Model file for the job. Use its own axes, mm. Face numbers are marked on the shaded views. A direction names the side the tool comes from. Round coordinates to 2 decimals unless told otherwise and drop trailing zeros. Loops run counter-clockwise (first coordinate to the right, second up) from the corner with the lowest first, then second, coordinate; pieces in that order, holes last. Notation, with made-up numbers: (-35, -7.75) -> (22, -7.75) arc R21 cw to (22, 30.25) -> close; hole circle Ø1 at (10, 75). An arc over 180 degrees is marked (long way). Use a Markdown table: item, result. Add a question column.
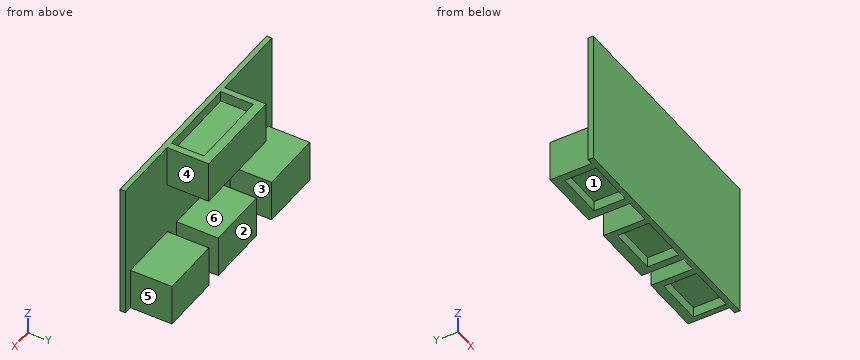
```python
from build123d import *

# Parameters (mm, degrees)
SKETCH1_W           = 23
SKETCH1_H           = 13
BOSS_EXTRUDE1_DEPTH = 0.5
SKETCH2_W           = 5.8
SKETCH2_H           = 4
SKETCH2_W_2         = 6
SKETCH2_W_3         = 9
BOSS_EXTRUDE2_DEPTH = 4
SKETCH3_W           = 4.624085026
SKETCH3_H           = 3.166867164
SKETCH3_W_2         = 4.718514666
SKETCH3_H_2         = 3.013327786
SKETCH3_W_3         = 4.580400568
CUT_EXTRUDE1_DEPTH  = 1
SKETCH4_W           = 7.748769295
SKETCH4_H           = 3.140290714
CUT_EXTRUDE2_DEPTH  = 1


with BuildPart() as part:
    # Sketch1 → Boss-Extrude1 (new body)
    with BuildSketch(Plane(origin=(0, 0, 0), x_dir=(1, 0, 0), z_dir=(0, 1, 0))):
        with Locations((1.517204559, 1.070232191)):
            Rectangle(SKETCH1_W, SKETCH1_H)
    extrude(amount=BOSS_EXTRUDE1_DEPTH)

    # Sketch2 → Boss-Extrude2 (add)
    with BuildSketch(Plane(origin=(0, 0.5, 0), x_dir=(1, 0, 0), z_dir=(0, 1, 0))):
        with Locations((9.339285907, 5.570232191)):
            Rectangle(SKETCH2_W, SKETCH2_H)
        with Locations((-6.403857402, 5.570232191)):
            Rectangle(SKETCH2_W_2, SKETCH2_H)
        with Locations((1.963830733, 5.570232191)):
            Rectangle(SKETCH2_W_2, SKETCH2_H)
        with Locations((1.962518624, -3.429767809)):
            Rectangle(SKETCH2_W_3, SKETCH2_H)
    extrude(amount=BOSS_EXTRUDE2_DEPTH)

    # Sketch3 → Cut-Extrude1 (cut)
    with BuildSketch(Plane(origin=(0, 0, -7.570232191), x_dir=(-1, 0, 0), z_dir=(0, 0, -1))):
        with Locations((-9.393748211, 2.083433582)):
            Rectangle(SKETCH3_W, SKETCH3_H)
        with Locations((-1.920682759, 2.006663893)):
            Rectangle(SKETCH3_W_2, SKETCH3_H_2)
        with Locations((6.437297708, 2.006663893)):
            Rectangle(SKETCH3_W_3, SKETCH3_H_2)
    extrude(amount=-CUT_EXTRUDE1_DEPTH, mode=Mode.SUBTRACT)

    # Sketch4 → Cut-Extrude2 (cut)
    with BuildSketch(Plane.XY.offset(5.429767809)):
        with Locations((1.929978032, 2.070145357)):
            Rectangle(SKETCH4_W, SKETCH4_H)
    extrude(amount=-CUT_EXTRUDE2_DEPTH, mode=Mode.SUBTRACT)


solid = part.part
```
1) Tool access for the marked faces 4, 5 and 6: list every direction of +Z, -Z, +X, -X, +Y, -Y with a clear straight run to the whole face (end or side of a thin tool).
2) Wall check: probe 1 along X at (y, z) = (1.25, -5.75); probe 2 along X at (y, z) = (1.35, -7); probe 3 along Z at (x, y) = (4, 0.75). Give the ranges that are in metal, low to high. Write a range as from..to.
3) Cut at D-D on z = 3.25. Write the cut outline in (x, y).
4) Pull direction Y, two halves, no side cores. Call the marked faces 1, 2 and 3: +Y half, -Y half, draft (parallel to the pull), parting line (faces both ways), or undercut.
5) Pin check, flat tips, straight feed: pin 1 Ø1.6 at (x, y) = (3, 2.5) entering from +Z; pin 2 Ø1.1 at (y, z) = (2, -7) entering from -X; pin 3 Ø0.5 at (y, z) = (1.5, -7) entering from +X. Stop position of each tip, or through.
6) Cut at C-C on y = 2.35. Count the separate pieces of the cut face and the enclosed holes in it, and give its area (3 significant figures).
7) Cut at B-B on x = 10.75. Write the cut outline in (y, z), and give its area (3 significant figures).
8) Cut at A-A on y = 4.05. Write the cut outline in (x, z).
Established:
| question | item | result |
|---|---|---|
| 1 | face 4 | +Z, +X, +Y |
| 1 | face 5 | +Z, -Z, +X, +Y |
| 1 | face 6 | +X, -X, +Y |
| 2 | probe 1 | x = -9.4..-3.4, -1.04..4.96, 6.44..12.24 |
| 2 | probe 2 | x = -9.4..-8.73, -4.15..-3.4, -1.04..-0.44, 4.28..4.96, 6.44..7.08, 11.71..12.24 |
| 2 | probe 3 | z = -6.57..-3.57, 1.43..4.43 |
| 3 | outline | (-9.98, 0) -> (13.02, 0) -> (13.02, 0.5) -> (6.46, 0.5) -> (6.46, 4.5) -> (-2.54, 4.5) -> (-2.54, 0.5) -> (-9.98, 0.5) -> close |
| 4 | face 1 | undercut |
| 4 | face 2 | +Y half |
| 4 | face 3 | draft |
| 5 | pin 1 | stops at z = 4.43 |
| 5 | pin 2 | stops at x = -9.4 |
| 5 | pin 3 | stops at x = 12.24 |
| 6 | separate pieces | 4 |
| 6 | enclosed holes | 0 |
| 6 | area | 85.5 mm^2 |
| 7 | outline | (0, -7.57) -> (0.5, -7.57) -> (0.5, -6.57) -> (3.67, -6.57) -> (3.67, -7.57) -> (4.5, -7.57) -> (4.5, -3.57) -> (0.5, -3.57) -> (0.5, 5.43) -> (0, 5.43) -> close |
| 7 | area | 19.3 mm^2 |
| 8 | outline | (-9.4, -7.57) -> (-3.4, -7.57) -> (-3.4, -3.57) -> (-9.4, -3.57) -> close; (-2.54, 1.43) -> (6.46, 1.43) -> (6.46, 5.43) -> (-2.54, 5.43) -> close; (-1.04, -7.57) -> (4.96, -7.57) -> (4.96, -3.57) -> (-1.04, -3.57) -> close; (6.44, -7.57) -> (12.24, -7.57) -> (12.24, -3.57) -> (6.44, -3.57) -> close |
